Autodesk Inventor part; units mm, degrees
ref_plane "YZ Plane" through (0, 0, 0) normal (1, 0, 0) x (0, 1, 0)
ref_plane "XZ Plane" through (0, 0, 0) normal (0, 1, 0) x (-1, 0, 0)
ref_plane "XY Plane" through (0, 0, 0) normal (0, 0, 1) x (1, 0, 0)
sketch "Sketch1" plane through (0, 0, 0) normal (1, 0, 0) x (0, 1, 0)
  circle A0 centre (0, 0) radius 3
  line L0 (3.6994, 0) -> (-3.9504, 0)
  line L1 (0, 0) -> (0, -4.1151)
  point P0 (0, -3)
  point P1 (3, 0)
  dimension "d0" = 6
revolve "Revolution1" add sketch "Sketch1" angle 360 about axis through (0, 0, 0) along (0, 0, -1) picked at (1.6828, -1.0574) contours A0 L1 L0
sketch "Sketch2" plane through (0, 0, 0) normal (0, 0, 1) x (1, 0, 0)
  circle A0 centre (0, 0) radius 3
extrude "Extrusion1" add sketch "Sketch2" along normal blind 3
sketch "Sketch3" plane through (0, 0, 3) normal (0, 0, 1) x (1, 0, 0)
  circle A0 centre (0, 0) radius 1.75
  dimension "d4" = 3.5
extrude "Extrusion2" cut sketch "Sketch3" against normal blind 4
thread "Thread1"
fillet "Fillet1" radius 0.5 1 edges at (-3, 0, 3)
fillet "Fillet2" radius 1 1 edges at (-1.75, 0, 3)
properties part number "torniquete"
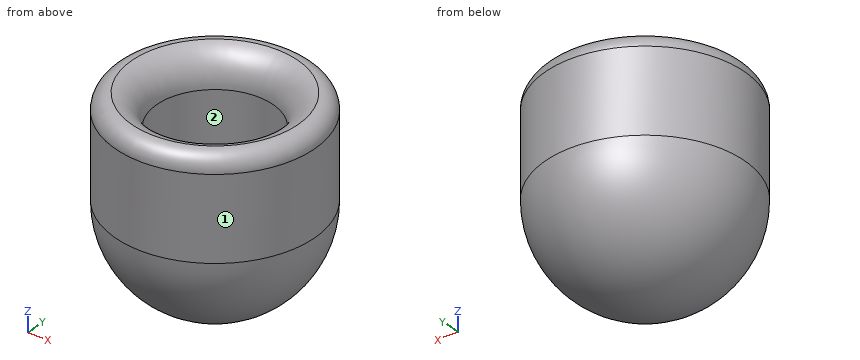
Source: CAD feature listing. Evaluate the final solid. Frame: model axes, mm. Face numbers are marked on the shaded views. Round coordinates to 2 decimals unless told otherwise and drop trailing zeros. Write each loop counter-clockwise with the first axis right and the second up, starting at its lowest first coordinate (ties: lowest second). Pieces come first, ordered by that corner, then holes. Notation, with made-up numbers: M 32,79.5 L 82,79.5 A23 ccw 82,117.5 Z; hole C 8,-29.5 d7. An arc over 180 degrees is marked long. Use CSV: the item, a comma, the result in double quotes. Start each with the question number.
Q1. Line query: line 1 (Y direction, x = 0, z = 0.55); line 2 (X direction, y = 1.05, z = 0.25); line 3 (X direction, y = 1.5, z = -0.05). Output: solid intervals per line, ascending. Write a range as from..to.
Q2. Cut plane A-A on x = 0. Output: boundary loops of the cut face in (y, z).
Q3. Cut plane C-C on z = 1.4. Output: boundary loops of the cut face in (x, y).
Q4. First-contact query: P1, Ø1, axis at x = 0.5, y = 0.5, coming from the +Z side. Flat tip, straight axial feed; report the tip coordinate or a pass-through.
Q5. Pull-direction query (Y, two-part tool) for the marked faces 1 and 2; classes: +Y half, -Y half, draft (parallel to the pull), parting line (faces both ways), or undercut.
Q6. Cut plane D-D on z = -1.25. Output: boundary loops of the cut face in (x, y).
Results found:
1,line 1,"-3..-1.75, 1.75..3"
1,line 2,"-2.81..-1.4, 1.4..2.81"
1,line 3,"-2.6..-0.9, 0.9..2.6"
2,outline,"M -3,0 A3 ccw 3,0 L 3,2.5 A0.5 ccw 2.5,3 A1 ccw 1.75,2.03 L 1.75,-1 L -1.75,-1 L -1.75,2.03 A1 ccw -2.5,3 A0.5 ccw -3,2.5 Z"
3,outline,"C 0,0 d6; hole C 0,0 d3.5"
4,P1,"z = -1"
5,face 1,"parting line"
5,face 2,"undercut"
6,outline,"C 0,0 d5.45"
